The listing builds one solid part. Answer for the finished solid, in the listing's coordinates (mm). Coordinates: 2 decimals unless noted, no trailing zeros. Order: outer loops, then holes, each group sorted by start corner. A loop starts at its lowest first (then second) coordinate and runs counter-clockwise, first axis right, second up.
```python
from build123d import *

# Parameters (mm, degrees)
F0_R     = 1.5
F1_DEPTH = 4


with BuildPart() as f1:
    # F0 (on Top) → F1 (new body)
    with BuildSketch(Plane.XY):
        with BuildLine():
            ThreePointArc((20.225759, -40.726859), (20.88342, -41.207836), (21.646246, -41.494115))
            Line((21.646246, -41.494115), (25.044904, -42.264138))
            Line((25.044904, -42.264138), (30.325992, -43.460657))
            ThreePointArc((30.325992, -43.460657), (31.363938, -43.61615), (32.391927, -43.404607))
            ThreePointArc((32.391927, -43.404607), (34.248228, -42.031919), (35.554256, -40.128129))
            ThreePointArc((35.554256, -40.128129), (35.729228, -39.093288), (35.537043, -38.061505))
            Line((35.537043, -38.061505), (34.154086, -32.826147))
            Line((34.154086, -32.826147), (33.264079, -29.456918))
            ThreePointArc((33.264079, -29.456918), (32.950942, -28.704719), (32.446956, -28.06452))
            Line((32.446956, -28.06452), (21.831277, -17.818679))
            ThreePointArc((21.831277, -17.818679), (21.047455, -16.969344), (20.366866, -16.035244))
            ThreePointArc((20.366866, -16.035244), (19.774372, -14.739531), (19.571381, -13.329314))
            Line((19.571381, -13.329314), (19.571381, 13.329314))
            ThreePointArc((19.571381, 13.329314), (19.774372, 14.739531), (20.366866, 16.035244))
            ThreePointArc((20.366866, 16.035244), (21.047455, 16.969344), (21.831277, 17.818679))
            Line((21.831277, 17.818679), (26.553101, 22.376))
            ThreePointArc((26.553101, 22.376), (27.441465, 23.354835), (28.192963, 24.442291))
            Line((28.192963, 24.442291), (32.873942, 32.276906))
            Line((32.873942, 32.276906), (18.454344, 40.892242))
            Line((18.454344, 40.892242), (16.119281, 36.984016))
            ThreePointArc((16.119281, 36.984016), (13.46563, 35.728384), (10.561704, 35.29746))
            Line((10.561704, 35.29746), (3.403735, 37.603494))
            ThreePointArc((3.403735, 37.603494), (0, 38.13824), (-3.403735, 37.603494))
            Line((-3.403735, 37.603494), (-10.561704, 35.29746))
            ThreePointArc((-10.561704, 35.29746), (-14.306504, 36.02511), (-17.506323, 38.102165))
            Line((-17.506323, 38.102165), (-19.467341, 39.994863))
            Line((-19.467341, 39.994863), (-20.225759, 40.726859))
            ThreePointArc((-20.225759, 40.726859), (-20.88342, 41.207836), (-21.646246, 41.494115))
            Line((-21.646246, 41.494115), (-25.044904, 42.264138))
            Line((-25.044904, 42.264138), (-30.325992, 43.460657))
            ThreePointArc((-30.325992, 43.460657), (-31.363938, 43.61615), (-32.391927, 43.404607))
            ThreePointArc((-32.391927, 43.404607), (-34.248228, 42.031919), (-35.554256, 40.128129))
            ThreePointArc((-35.554256, 40.128129), (-35.729228, 39.093288), (-35.537043, 38.061505))
            Line((-35.537043, 38.061505), (-34.154086, 32.826147))
            Line((-34.154086, 32.826147), (-33.264079, 29.456918))
            ThreePointArc((-33.264079, 29.456918), (-32.950942, 28.704719), (-32.446956, 28.06452))
            Line((-32.446956, 28.06452), (-21.831277, 17.818679))
            ThreePointArc((-21.831277, 17.818679), (-21.047455, 16.969344), (-20.366866, 16.035244))
            ThreePointArc((-20.366866, 16.035244), (-19.774372, 14.739531), (-19.571381, 13.329314))
            Line((-19.571381, 13.329314), (-19.571381, -13.329314))
            ThreePointArc((-19.571381, -13.329314), (-19.774372, -14.739531), (-20.366866, -16.035244))
            ThreePointArc((-20.366866, -16.035244), (-21.047455, -16.969344), (-21.831277, -17.818679))
            Line((-21.831277, -17.818679), (-32.446956, -28.06452))
            ThreePointArc((-32.446956, -28.06452), (-32.950942, -28.704719), (-33.264079, -29.456918))
            Line((-33.264079, -29.456918), (-34.154086, -32.826147))
            Line((-34.154086, -32.826147), (-35.537043, -38.061505))
            ThreePointArc((-35.537043, -38.061505), (-35.729228, -39.093288), (-35.554256, -40.128129))
            ThreePointArc((-35.554256, -40.128129), (-34.248228, -42.031919), (-32.391927, -43.404607))
            ThreePointArc((-32.391927, -43.404607), (-31.363938, -43.61615), (-30.325992, -43.460657))
            Line((-30.325992, -43.460657), (-25.044904, -42.264138))
            Line((-25.044904, -42.264138), (-21.646246, -41.494115))
            ThreePointArc((-21.646246, -41.494115), (-20.88342, -41.207836), (-20.225759, -40.726859))
            Line((-20.225759, -40.726859), (-19.467341, -39.994863))
            Line((-19.467341, -39.994863), (-17.506323, -38.102165))
            ThreePointArc((-17.506323, -38.102165), (-14.306504, -36.02511), (-10.561704, -35.29746))
            Line((-10.561704, -35.29746), (10.561704, -35.29746))
            ThreePointArc((10.561704, -35.29746), (14.306504, -36.02511), (17.506323, -38.102165))
            Line((17.506323, -38.102165), (19.467341, -39.994863))
            Line((19.467341, -39.994863), (20.225759, -40.726859))
        make_face()
        with Locations((-28.491992, -36.476224)):
            Circle(F0_R, mode=Mode.SUBTRACT)
        with Locations((-22.735756, -30.920528)):
            Circle(F0_R, mode=Mode.SUBTRACT)
        with Locations((28.491992, -36.476224)):
            Circle(F0_R, mode=Mode.SUBTRACT)
        with Locations((22.735756, -30.920528)):
            Circle(F0_R, mode=Mode.SUBTRACT)
        with Locations((-22.735756, 30.920528)):
            Circle(F0_R, mode=Mode.SUBTRACT)
        with Locations((-28.491992, 36.476224)):
            Circle(F0_R, mode=Mode.SUBTRACT)
    extrude(amount=F1_DEPTH)


solid = f1.part
```
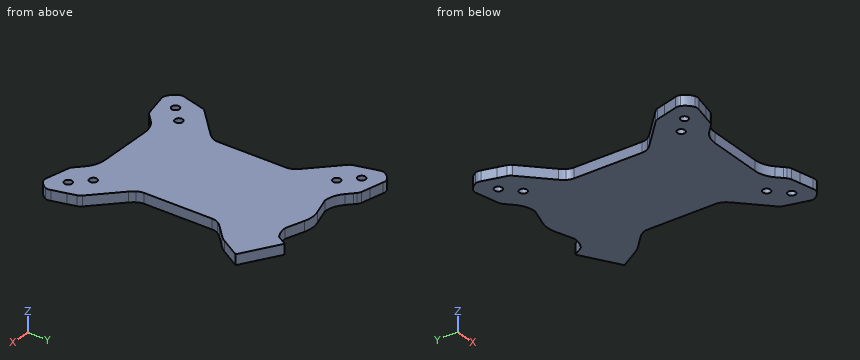
(1) Each of these flat-tipped pins is pushed along its axis until it touches: pin 1 Ø1 at (x, z) = (2.5, 0.5) entering from +Y; pin 2 Ø2 at (x, z) = (-1, 2.5) entering from -Y. Where does it stop, or does it pass through?
(2) Consider line 1 (Y direction, x = -23.5, z = 0.85); line 2 (Y direction, x = 29, z = 3.2); line 3 (Y direction, x = 28.5, z = 1.05). Determine where each line is inside the solid, lowest interval first.
(3) Find section C-C (z = 2.95). Give the number of separate pieces and of enclosed holes in the cut face, and give its area (3 significant figures).
(4) Find section B-B (x = 5). Write down the section's boundary in (y, z), and give its area (3 significant figures).
(5) Find section A-A (y = -10). Write down the section's boundary in (x, z), and give its area (3 significant figures).
Findings below:
1. pin 1: stops at y = 37.96
1. pin 2: stops at y = -35.3
2. line 1: y = -41.91 to -32.21, -29.63 to -19.43, 19.43 to 29.63, 32.21 to 41.91
2. line 2: y = -43.16 to -37.89, -35.06 to -24.74, 25.79 to 34.59
2. line 3: y = -43.05 to -37.98, -34.98 to -24.26, 24.96 to 34.89
3. separate pieces: 1
3. enclosed holes: 6
3. area: 3,880 mm2
4. outline: (-35.3, 0) - (37.09, 0) - (37.09, 4) - (-35.3, 4) - close
4. area: 290 mm2
5. outline: (-19.57, 0) - (19.57, 0) - (19.57, 4) - (-19.57, 4) - close
5. area: 157 mm2
